```python
from build123d import *

# Parameters (mm, degrees)
BOSS_EXTRUDE1_DEPTH = 500
SKETCH2_R           = 2.75
CUT_EXTRUDE1_DEPTH  = 502.554026994


with BuildPart() as part:
    # Sketch1 → Boss-Extrude1 (new body)
    with BuildSketch(Plane.XY):
        with BuildLine():
            Line((-21.620406895, 0), (18.379593105, 0))
            Line((18.379593105, 0), (18.379593105, 5))
            Line((18.379593105, 5), (9.152634797, 5))
            Line((9.152634797, 5), (9.152634797, 10))
            Line((9.152634797, 10), (2.379593105, 18.07179677))
            ThreePointArc((2.379593105, 18.07179677), (-1.620406895, 33), (-5.620406895, 18.07179677))
            Line((-5.620406895, 18.07179677), (-12.393448588, 10))
            Line((-12.393448588, 10), (-12.393448588, 5))
            Line((-12.393448588, 5), (-21.620406895, 5))
            Line((-21.620406895, 5), (-21.620406895, 0))
        make_face()
    extrude(amount=BOSS_EXTRUDE1_DEPTH)

    # Sketch2 → Cut-Extrude1 (cut, through all)
    with BuildSketch(Plane(origin=(0, 0, 0), x_dir=(1, 0, 0), z_dir=(0, 1, 0))):
        with Locations(Location((-16.620406895, -475, 0), (0, 0, 90))):
            Circle(SKETCH2_R)
        with Locations(Location((13.379593105, -475, 0), (0, 0, 90))):
            Circle(SKETCH2_R)
        with Locations(Location((-16.620406895, -325, 0), (0, 0, 90))):
            Circle(SKETCH2_R)
        with Locations(Location((13.379593105, -325, 0), (0, 0, 90))):
            Circle(SKETCH2_R)
        with Locations(Location((-16.620406895, -175, 0), (0, 0, 90))):
            Circle(SKETCH2_R)
        with Locations(Location((13.379593105, -175, 0), (0, 0, 90))):
            Circle(SKETCH2_R)
        with Locations(Location((-16.620406895, -25, 0), (0, 0, 90))):
            Circle(SKETCH2_R)
        with Locations(Location((13.379593105, -25, 0), (0, 0, 90))):
            Circle(SKETCH2_R)
    extrude(amount=CUT_EXTRUDE1_DEPTH, mode=Mode.SUBTRACT)


solid = part.part
```
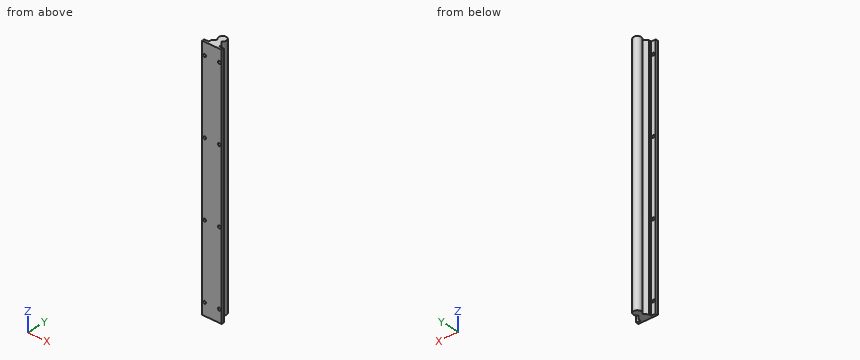
Input: part model. Units: mm. Frame: model coordinates. Coordinates: 2 decimals unless noted, no trailing zeros. Loops run counter-clockwise (first coordinate to the right, second up) from the corner with the lowest first, then second, coordinate; pieces in that order, holes last. Notation, with made-up numbers: M 89.25,35.25 L 104.25,35.25 A22 ccw 104.25,53.25 Z; hole C 28.5,70.5 d10. An arc over 180 degrees is marked long. Answer in a Markdown table with one row per item.
1. Section B-B, the plane y = 25. Output: boundary loops of the cut face in (x, z).
Response:
| item | result |
|---|---|
| outline | M -9.62,0 L 6.38,0 L 6.38,500 L -9.62,500 Z |
2. First-contact query: pin 1 (10 mm diameter, centred on x = 15.5, z = 231.5, fed in from +Y); pin 2 (4 mm diameter, centred on y = 7.5, z = 303.5, fed in from -X); pin 3 (5 mm diameter, centred on y = 20.5, z = 232, fed in from -X); pin 4 (1.5 mm diameter, centred on x = -14.5, y = 11.5, fed in from -Z). Flat tips, straight axial feed; report the tip coordinate or a pass-through.
Response:
| item | result |
|---|---|
| pin 1 | stops at y = 5 |
| pin 2 | stops at x = -12.39 |
| pin 3 | stops at x = -9.37 |
| pin 4 | passes through |
3. Material intervals for line 1 (X direction, y = 3.8, z = 175); line 2 (X direction, y = 7, z = 67.5); line 3 (X direction, y = 24, z = 394), sorted ascending.
Response:
| item | result |
|---|---|
| line 1 | x = -21.62 to -19.37, -13.87 to 10.63, 16.13 to 18.38 |
| line 2 | x = -12.39 to 9.15 |
| line 3 | x = -9.56 to 6.32 |
4. Section A-A, the plane z = 243. Output: boundary loops of the cut face in (x, y), then the cut area to 3 significant figures.
Response:
| item | result |
|---|---|
| outline | M -21.62,0 L 18.38,0 L 18.38,5 L 9.15,5 L 9.15,10 L 2.38,18.07 A8 ccw long -5.62,18.07 L -12.39,10 L -12.39,5 L -21.62,5 Z |
| area | 622 mm2 |
